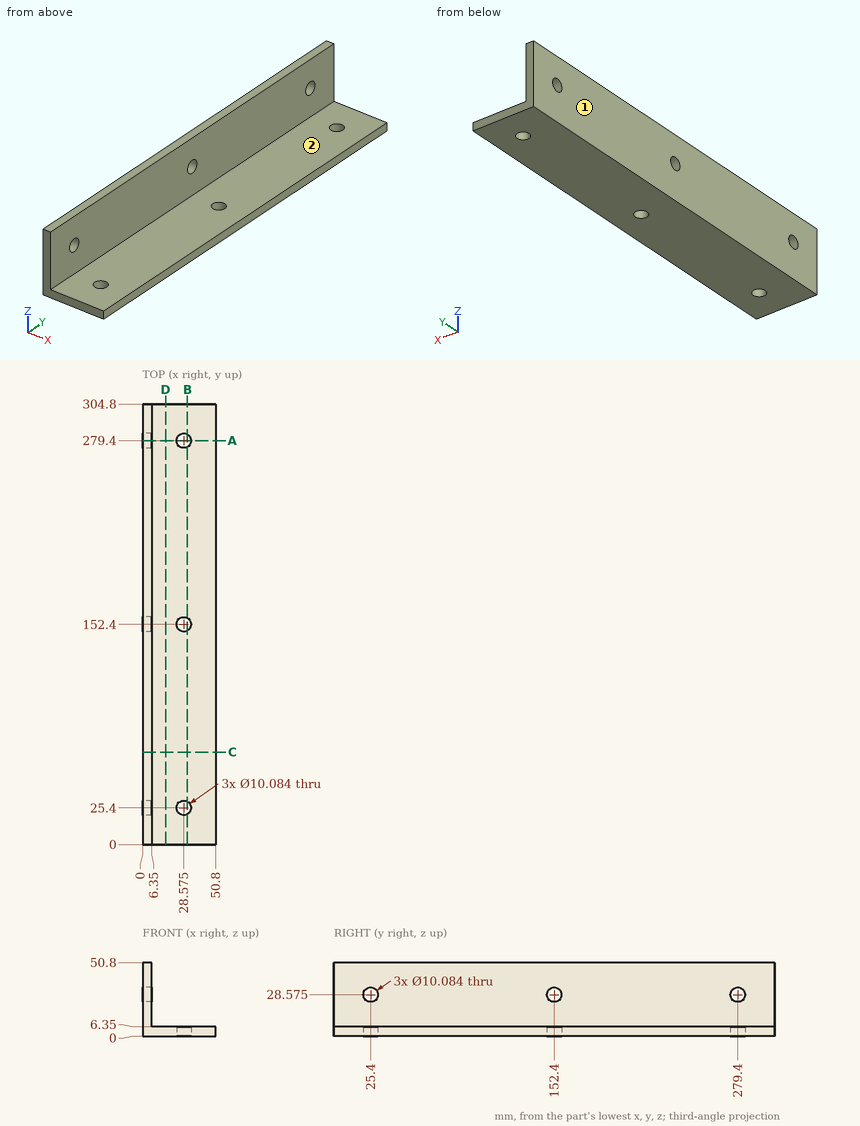
Job drawing, mm, ordinate dimensions from the low corner. One solid piece. A direction names the side the tool comes from. Round coordinates to 2 decimals unless told otherwise and drop trailing zeros. Order: outer loops, then holes, each group sorted by start corner. A loop starts at its lowest first (then second) coordinate and runs counter-clockwise, first axis right, second up. Notation, with made-up numbers: (10, 55) - (69, 55) arc R17 cw to (69, 66) - close; hole circle Ø8 at (42.25, 89). An arc over 180 degrees is marked (long way). Use CSV: the item, a comma, the result in double quotes. Start each with the question number.
1) Saw through at D-D (x = 16). List the corners of the cut face in (y, z).
2) Saw through at B-B (x = 31). List the corners of the cut face in (y, z), and give its area (3 significant figures).
3) Saw through at A-A (y = 279.4). List the corners of the cut face in (x, z), and give its area (3 significant figures).
4) Wall check: L1, parallel to Z at x = 4.5, y = 25.4; L2, parallel to X at y = 279, z = 2; L3, parallel to X at y = 20.5, z = 41. Give the ranges that are in metal, low to high. Write a range as [from, to].
5) Pin check, flat tips, straight feed: pin 1 Ø6 at (x, y) = (28.575, 152.4) entering from -Z; pin 2 Ø11.5 at (y, z) = (152.4, 28.575) entering from +X; pin 3 Ø3 at (x, y) = (11, 247) entering from +Z. Stop position of each tip, or through.
6) Tool access for the marked faces 1 and 2: list every direction of +Z, -Z, +X, -X, +Y, -Y with a clear straight run to the whole face (end or side of a thin tool).
7) Saw through at C-C (y = 64). List the corners of the cut face in (x, z).
Values follow:
1,outline,"(0, 0) - (304.8, 0) - (304.8, 6.35) - (0, 6.35) - close"
2,outline,"(0, 0) - (20.98, 0) - (20.98, 6.35) - (0, 6.35) - close; (29.82, 0) - (147.98, 0) - (147.98, 6.35) - (29.82, 6.35) - close; (156.82, 0) - (274.98, 0) - (274.98, 6.35) - (156.82, 6.35) - close; (283.82, 0) - (304.8, 0) - (304.8, 6.35) - (283.82, 6.35) - close"
2,area,"1,770 mm2"
3,outline,"(0, 0) - (23.53, 0) - (23.53, 6.35) - (6.35, 6.35) - (6.35, 23.53) - (0, 23.53) - close; (0, 33.62) - (6.35, 33.62) - (6.35, 50.8) - (0, 50.8) - close; (33.62, 0) - (50.8, 0) - (50.8, 6.35) - (33.62, 6.35) - close"
3,area,"477 mm2"
4,L1,"z = [0, 23.53], [33.62, 50.8]"
4,L2,"x = [0, 23.55], [33.6, 50.8]"
4,L3,"x = [0, 6.35]"
5,pin 1,"passes through"
5,pin 2,"stops at x = 6.35"
5,pin 3,"stops at z = 6.35"
6,face 1,"+Z, -Z, -X, +Y, -Y"
6,face 2,"+Z, +X, +Y, -Y"
7,outline,"(0, 0) - (50.8, 0) - (50.8, 6.35) - (6.35, 6.35) - (6.35, 50.8) - (0, 50.8) - close"
